Geometry: final body of the model. Coordinates: model frame, mm. A direction names the side the tool comes from. Round coordinates to 2 decimals unless told otherwise and drop trailing zeros. Order: outer loops, then holes, each group sorted by start corner. A loop starts at its lowest first (then second) coordinate and runs counter-clockwise, first axis right, second up. Notation, with made-up numbers: (34, 9) - (82, 9) arc R23 cw to (82, 22) - close; hole circle Ø4 at (81, 65). An arc over 180 degrees is marked (long way). Put each result on its own line as item: value. Start each with the question number.
(1) Section C-C (z = 24.9). Output: boundary loops of the cut face in (x, y) (3 decimals), and give its area (3 significant figures).
(2) Section A-A (x = 0). Output: boundary loops of the cut face in (y, z) (3 decimals), and give its area (3 significant figures).
(3) Section B-B (y = 10.5). Output: boundary loops of the cut face in (x, z), and give its area (3 significant figures).
(4) Material intervals for L1, parallel to Y at x = 18.5, z = 24.5; L2, parallel to Y at x = -46, z = 25.55 (3 decimals); L3, parallel to X at y = 0, z = 25.85, sorted ascending. Write a range as [from, to].
(5) Section D-D (x = -15.5). Output: boundary loops of the cut face in (y, z) (3 decimals), and give its area (3 significant figures).
(6) Pull-direction query (Y, two-part tool) for faces 1 (the face through (5.825, 6, 25)), 2 (the face through (-3, 18.324, 25)), 3 (the face through (-11.025, 14, 25)); classes: released by +Y, released by -Y, zero draft, split by the parting line, or undercut.
(7) Access query for faces 4 (the face through (4.8, 2.01, 25.02)), 5 (the face through (-30, 8.775, 25)), 6 (the face through (-11.025, -11, 25)). Directions: +Z, -Z, +X, -X, +Y, -Y. A direction counts if a zero-diameter tool reaches every point of the face in a straight line with its end or side. Return the directions, or none.
(8) Pin query (flat end, axial travel): P1, Ø0.8, axis at y = -7, z = 24.5, coming from the -X side; P2, Ø0.8, axis at y = 24.5, z = 25, coming from the -X side; P3, Ø5.5, axis at x = 0, y = 0, coming from the +Z side. Return the tip coordinate at first contact, or that it passes through.
from build123d import *

# Parameters (mm, degrees)
F0_W     = 11.65
F0_H     = 23.75
F1_DEPTH = 20.4
F3_DEPTH = 6
F5_START = -0.8
F4_W     = 11.65
F4_H     = 4.2
F5_DEPTH = 2
F6_R     = 0.5
F7_R     = 1
F8_R     = 1.4
F9_DEPTH = 2.8
F10_R    = 4


# Not quite as in the source:
# - a feature names something its author has since deleted; it is built from what else it names


with BuildPart() as f1:
    # F0 (on Top) → F1 (new body)
    with BuildSketch(Plane.XY):
        Rectangle(F0_W, F0_H)
    extrude(amount=F1_DEPTH)

    # F2 (on face) → F3 (join)
    with BuildSketch(Plane.XY.offset(20.4)):
        with BuildLine():
            Line((5.825, 3.9640955299), (5.825, 7.5859044701))
            ThreePointArc((5.825, 7.5859044701), (0, 11.875), (-5.825, 7.5859044701))
            Line((-5.825, 7.5859044701), (-5.825, 3.9640955299))
            ThreePointArc((-5.825, 3.9640955299), (-4.7781429098, 1.9829886164), (-3.0865775367, 0.5135326087))
            ThreePointArc((-3.0865775367, 0.5135326087), (0, -3.1), (3.0865775367, 0.5135326087))
            ThreePointArc((3.0865775367, 0.5135326087), (4.7781429098, 1.9829886164), (5.825, 3.9640955299))
        make_face()
    extrude(amount=F3_DEPTH)

    # F4 (on face) → F5 (join)
    with BuildSketch(Plane.XY.offset(20.4).offset(F5_START)):
        with Locations((0, -13.975)):
            Rectangle(F4_W, F4_H)
        with Locations((0, 13.975)):
            Rectangle(F4_W, F4_H)
    extrude(amount=-F5_DEPTH)

    # F6
    f6_edges = [f1.edges().sort_by_distance(p)[0] for p in [
        (5.825, 11.875, 8.8),
        (5.825, -11.875, 8.8),
        (-5.825, -11.875, 8.8),
        (-5.825, 11.875, 8.8),
    ]]
    fillet(f6_edges, radius=F6_R)

    # F7
    f7_edges = [f1.edges().sort_by_distance(p)[0] for p in [
        (-5.825, 16.075, 18.6),
        (5.825, 16.075, 18.6),
        (5.825, -16.075, 18.6),
        (-5.825, -16.075, 18.6),
    ]]
    fillet(f7_edges, radius=F7_R)


with BuildPart() as f9:
    # F8 (on face) → F9 (new body)
    with BuildSketch(Plane.XY.offset(26.4)):
        with BuildLine():
            Line((22.5, -26), (22.5, 30))
            Line((22.5, 30), (4.6129450202, 30))
            Line((4.6129450202, 30), (4.6129450202, 21.3236394078))
            ThreePointArc((4.6129450202, 21.3236394078), (3.7342653638, 19.2023190642), (1.6129450202, 18.3236394078))
            Line((1.6129450202, 18.3236394078), (-8.0251465812, 18.3236394078))
            ThreePointArc((-8.0251465812, 18.3236394078), (-10.1464669248, 17.4449597513), (-11.0251465812, 15.3236394078))
            Line((-11.0251465812, 15.3236394078), (-11.0251465812, 11.775))
            ThreePointArc((-11.0251465812, 11.775), (-11.9038262377, 9.6536796564), (-14.0251465812, 8.775))
            Line((-14.0251465812, 8.775), (-46, 8.775))
            ThreePointArc((-46, 8.775), (-49, 5.775), (-46, 2.775))
            Line((-46, 2.775), (-14.0251465812, 2.775))
            ThreePointArc((-14.0251465812, 2.775), (-11.9038262377, 1.8963203436), (-11.0251465812, -0.225))
            Line((-11.0251465812, -0.225), (-11.0251465812, -15.0673655123))
            Line((-11.0251465812, -15.0673655123), (-11.0251465812, -26))
            Line((-11.0251465812, -26), (22.5, -26))
        make_face()
        with Locations((-7.0251465812, -22)):
            Circle(F8_R, mode=Mode.SUBTRACT)
        with Locations((18.5, -22)):
            Circle(F8_R, mode=Mode.SUBTRACT)
        with Locations((-46, 5.775)):
            Circle(F8_R, mode=Mode.SUBTRACT)
        with BuildLine():
            ThreePointArc((5.825, 3.9640955299), (4.7781429098, 1.9829886164), (3.0865775367, 0.5135326087))
            ThreePointArc((3.0865775367, 0.5135326087), (0, -3.1290056936), (-3.0865775367, 0.5135326087))
            ThreePointArc((-3.0865775367, 0.5135326087), (-4.7781429098, 1.9829886164), (-5.825, 3.9640955299))
            Line((-5.825, 3.9640955299), (-5.825, 7.5859044701))
            ThreePointArc((-5.825, 7.5859044701), (0, 11.875), (5.825, 7.5859044701))
            Line((5.825, 7.5859044701), (5.825, 3.9640955299))
        make_face(mode=Mode.SUBTRACT)
        with Locations((18.5, 26)):
            Circle(F8_R, mode=Mode.SUBTRACT)
    extrude(amount=-F9_DEPTH)

    # F10
    f10_edges = [f9.edges().sort_by_distance(p)[0] for p in [
        (22.5, 30, 25),
        (-11.025147, -26, 25),
        (22.5, -26, 25),
        (4.612945, 30, 25),
    ]]
    fillet(f10_edges, radius=F10_R)


with BuildPart() as f11_1:
    # F11: copy of F9
    add(f9.part)


solid = f9.part
Checks:
1. outline: (-46, 2.775) - (-14.025, 2.775) arc R3 cw to (-11.025, -0.225) - (-11.025, -22) arc R4 ccw to (-7.025, -26) - (18.5, -26) arc R4 ccw to (22.5, -22) - (22.5, 26) arc R4 ccw to (18.5, 30) - (8.613, 30) arc R4 ccw to (4.613, 26) - (4.613, 21.324) arc R3 cw to (1.613, 18.324) - (-8.025, 18.324) arc R3 ccw to (-11.025, 15.324) - (-11.025, 11.775) arc R3 cw to (-14.025, 8.775) - (-46, 8.775) arc R3 ccw to start; hole circle Ø2.8 at (-46, 5.775); hole circle Ø2.8 at (-7.025, -22); hole (-5.825, 3.964) arc R6.1 ccw to (-3.087, 0.514) arc R3.129 ccw (long way) to (3.087, 0.514) arc R6.1 ccw to (5.825, 3.964) - (5.825, 7.586) arc R6.1 ccw to (-5.825, 7.586) - close; hole circle Ø2.8 at (18.5, -22); hole circle Ø2.8 at (18.5, 26)
1. area: 1,750 mm²
2. outline: (-26, 23.6) - (-3.129, 23.6) - (-3.129, 26.4) - (-26, 26.4) - close; (11.875, 23.6) - (18.324, 23.6) - (18.324, 26.4) - (11.875, 26.4) - close
2. area: 82.1 mm²
3. outline: (-11.31, 23.6) - (-3.86, 23.6) - (-3.86, 26.4) - (-11.31, 26.4) - close; (3.86, 23.6) - (22.5, 23.6) - (22.5, 26.4) - (3.86, 26.4) - close
3. area: 73.1 mm²
4. L1: y = [-26, -23.4], [-20.6, 24.6], [27.4, 30]
4. L2: y = [2.775, 4.375], [7.175, 8.775]
4. L3: x = [-11.03, -3.13], [3.13, 22.5]
5. outline: (2.775, 23.6) - (8.775, 23.6) - (8.775, 26.4) - (2.775, 26.4) - close
5. area: 16.8 mm²
6. face 1: undercut
6. face 2: released by +Y
6. face 3: zero draft
7. face 4: +Z, -Z
7. face 5: +Z, -Z, -X, +Y
7. face 6: +Z, -Z, -X, -Y
8. P1: stops at x = -11.03
8. P2: stops at x = 4.61
8. P3: passes through
